from build123d import *

# Parameters (mm, degrees)
F1_DEPTH     = 22
F3_DEPTH     = 25
F4_DEPTH     = 11
F5_R         = 1.75
F6_DEPTH     = 20
F7_T1_DEPTH  = 22
F7_T6_DEPTH  = 22
F7_S7_R      = 1.75
F7_T8_DEPTH  = 14
F7_S9_R      = 1.75
F7_T10_DEPTH = 14


# Not quite as in the source:
# - a fillet or chamfer that OpenCascade refuses, or shapes differently, is made with other operations: its cross-section is extruded or revolved along the edge and cut away or added
# - after a boolean that leaves OpenCascade's solid faulty, fix() repairs it


with BuildPart() as f1:
    # F0 (on Right) → F1 (new body)
    with BuildSketch(Plane.YZ):
        with BuildLine():
            ThreePointArc((-20.9761769634, 1), (0, 21), (20.9761769634, 1))
            Line((20.9761769634, 1), (35.9761769634, 1))
            Line((35.9761769634, 1), (35.9761769634, 23))
            Line((35.9761769634, 23), (-36, 23))
            Line((-36, 23), (-36, 1))
            Line((-36, 1), (-20.9761769634, 1))
        make_face()
        with BuildLine():
            ThreePointArc((-18.973665961, -1), (-18.9934153493, -0.5001733404), (-19, 0))
            Line((-19, 0), (-21, 0))
            ThreePointArc((-21, 0), (-20.9940433961, -0.5001418641), (-20.9761769634, -1))
            Line((-20.9761769634, -1), (-18.973665961, -1))
        make_face()
        with BuildLine():
            ThreePointArc((18.973665961, 1), (1, -18.973665961), (-18.973665961, -1))
            Line((-18.973665961, -1), (-20.9761769634, -1))
            ThreePointArc((-20.9761769634, -1), (1, -20.9761769634), (20.9761769634, 1))
            Line((20.9761769634, 1), (18.973665961, 1))
        make_face()
        with BuildLine():
            ThreePointArc((-18.973665961, 1), (0, 19), (18.973665961, 1))
            Line((18.973665961, 1), (20.9761769634, 1))
            ThreePointArc((20.9761769634, 1), (0, 21), (-20.9761769634, 1))
            Line((-20.9761769634, 1), (-18.973665961, 1))
        make_face()
        with BuildLine():
            ThreePointArc((-20.9761769634, -1), (-20.9940433961, -0.5001418641), (-21, 0))
            Line((-21, 0), (-36, 0))
            Line((-36, 0), (-36, -1))
            Line((-36, -1), (-20.9761769634, -1))
        make_face()
    extrude(amount=F1_DEPTH)

    # F2 (on face) → F3 (cut)
    with BuildSketch(Plane.XY.offset(23)):
        with BuildLine():
            ThreePointArc((4.25, -24.9799919936), (6, -26.7299919936), (7.75, -24.9799919936))
            Line((7.75, -24.9799919936), (6, -24.9799919936))
            Line((6, -24.9799919936), (4.25, -24.9799919936))
        make_face()
        with BuildLine():
            Line((6, -24.9799919936), (5.93, -23.231392554))
            ThreePointArc((5.93, -23.231392554), (4.7380570536, -23.7675564283), (4.25, -24.9799919936))
            Line((4.25, -24.9799919936), (6, -24.9799919936))
        make_face()
        with BuildLine():
            Line((6, -24.9799919936), (7.75, -24.9799919936))
            ThreePointArc((7.75, -24.9799919936), (7.2124355653, -23.7180490472), (5.93, -23.231392554))
            Line((5.93, -23.231392554), (6, -24.9799919936))
        make_face()
        with BuildLine():
            ThreePointArc((17.75, -24.9799919936), (16, -23.2299919936), (14.25, -24.9799919936))
            ThreePointArc((14.25, -24.9799919936), (16, -26.7299919936), (17.75, -24.9799919936))
        make_face()
    extrude(amount=-F3_DEPTH, mode=Mode.SUBTRACT)

    # F2 (on face) → F4 (cut)
    with BuildSketch(Plane.XY.offset(23)):
        with BuildLine():
            Line((9, -24.9799919936), (7.75, -24.9799919936))
            ThreePointArc((7.75, -24.9799919936), (6, -26.7299919936), (4.25, -24.9799919936))
            Line((4.25, -24.9799919936), (3, -24.9799919936))
            ThreePointArc((3, -24.9799919936), (6, -27.9799919936), (9, -24.9799919936))
        make_face()
        with BuildLine():
            ThreePointArc((4.25, -24.9799919936), (4.7380570536, -23.7675564283), (5.93, -23.231392554))
            Line((5.93, -23.231392554), (5.88, -21.9823929544))
            ThreePointArc((5.88, -21.9823929544), (3.8366692347, -22.9015310245), (3, -24.9799919936))
            Line((3, -24.9799919936), (4.25, -24.9799919936))
        make_face()
        with BuildLine():
            ThreePointArc((5.93, -23.231392554), (7.2124355653, -23.7180490472), (7.75, -24.9799919936))
            Line((7.75, -24.9799919936), (9, -24.9799919936))
            ThreePointArc((9, -24.9799919936), (8.0784609691, -22.8166612283), (5.88, -21.9823929544))
            Line((5.88, -21.9823929544), (5.93, -23.231392554))
        make_face()
        with BuildLine():
            ThreePointArc((19, -24.9799919936), (16, -21.9799919936), (13, -24.9799919936))
            ThreePointArc((13, -24.9799919936), (16, -27.9799919936), (19, -24.9799919936))
        make_face()
        with BuildLine():
            ThreePointArc((17.75, -24.9799919936), (16, -26.7299919936), (14.25, -24.9799919936))
            ThreePointArc((14.25, -24.9799919936), (16, -23.2299919936), (17.75, -24.9799919936))
        make_face(mode=Mode.SUBTRACT)
    extrude(amount=-F4_DEPTH, mode=Mode.SUBTRACT)

    # F7: fillet of radius 10 on 2 edges, made by hand

    # F7_s2 → F7_t1 (join)
    with BuildSketch(Plane.YZ):
        with BuildLine():
            ThreePointArc((29.6647939484, 1), (23.7079599766, -0.967806711), (20.095505578, -6.0967741935))
            ThreePointArc((20.095505578, -6.0967741935), (20.8401494161, -2.5861500957), (20.9761769634, 1))
            Line((20.9761769634, 1), (29.6647939484, 1))
        make_face()
    extrude(amount=F7_T1_DEPTH)


with BuildPart() as f6:
    # F5 (on face) → F6 (new body)
    with BuildSketch(Plane(origin=(0, 0, -1), x_dir=(1, 0, 0), z_dir=(0, 0, -1))):
        Polygon((19.897114317, 27.2299919936), (16, 29.4799919936), (12.102885683, 27.2299919936), (12.102885683, 22.7299919936), (15.1405824223, 20.9761769634), (16.8594175777, 20.9761769634), (19.897114317, 22.7299919936), align=None)
        with Locations((16, 24.9799919936)):
            Circle(F5_R, mode=Mode.SUBTRACT)
    extrude(amount=F6_DEPTH)


with BuildPart() as f6b:
    # F5 (on face) → F6, piece 2 (new body)
    with BuildSketch(Plane(origin=(0, 0, -1), x_dir=(1, 0, 0), z_dir=(0, 0, -1))):
        Polygon((5.1405824223, 20.9761769634), (6.8594175777, 20.9761769634), (9.897114317, 22.7299919936), (9.897114317, 27.2299919936), (6, 29.4799919936), (2.102885683, 27.2299919936), (2.102885683, 22.7299919936), align=None)
        with Locations((6, 24.9799919936)):
            Circle(F5_R, mode=Mode.SUBTRACT)
    extrude(amount=F6_DEPTH)


with BuildPart() as f7_tool4:
    # F7_s5 → F7_t6 (new body)
    with BuildSketch(Plane.YZ):
        with BuildLine():
            ThreePointArc((-28.9827534924, -1), (-23.3031351499, -2.7694510825), (-19.6334781723, -7.4516129032))
            ThreePointArc((-19.6334781723, -7.4516129032), (-20.5594710492, -4.2788024233), (-20.9761769634, -1))
            Line((-20.9761769634, -1), (-28.9827534924, -1))
        make_face()
    extrude(amount=F7_T6_DEPTH)

    # F7_s7 → F7_t8 (cut, symmetric)
    with BuildSketch(Plane.XY.offset(-4.2)):
        with Locations((16, -24.9799919936)):
            Circle(F7_S7_R)
    extrude(amount=F7_T8_DEPTH, both=True, mode=Mode.SUBTRACT)

    # F7_s9 → F7_t10 (cut, symmetric)
    with BuildSketch(Plane.XY.offset(-4.2)):
        with Locations((6, -24.9799919936)):
            Circle(F7_S9_R)
    extrude(amount=F7_T10_DEPTH, both=True, mode=Mode.SUBTRACT)


with BuildPart() as f1_1:
    add(f1.part)

    # F7_t3: union F7_tool4
    add(f7_tool4.part)

    # F8: cut F6, F6b
    add(f6.part, mode=Mode.SUBTRACT)
    add(f6b.part, mode=Mode.SUBTRACT)

    add(f1_1.part.fix(), mode=Mode.REPLACE)


solid = f1_1.part
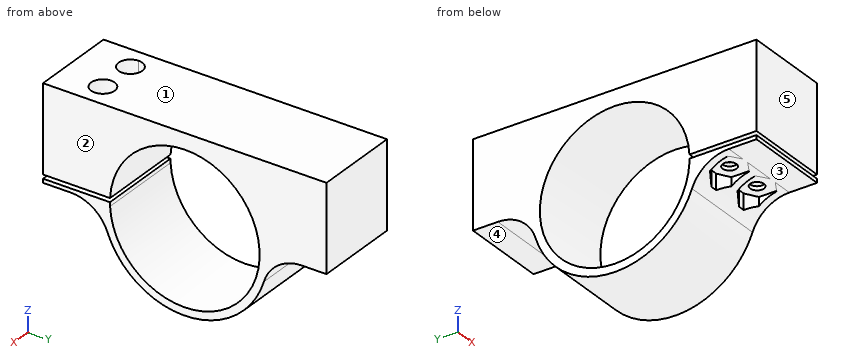
Input: part model. Units: mm. Frame: model coordinates. Face numbers are marked on the shaded views. A direction names the side the tool comes from. Coordinates: 2 decimals unless noted, no trailing zeros. Loops run counter-clockwise (first coordinate to the right, second up) from the corner with the lowest first, then second, coordinate; pieces in that order, holes last.
(1) Section B-B on x = 16. Return the cut outline in (y, z).
(2) First-contact query: pin 1 Ø3 at (x, y) = (15.5, -26) entering from +Z; pin 2 Ø1 at (x, y) = (7, -13.5) entering from -Z; pin 3 Ø7 at (x, y) = (15.5, 32) entering from -Z; pin 4 Ø2 at (x, y) = (16, -24.98) entering from +Z. Flat tips, straight axial feed; report the tip coordinate or a pass-through.
(3) Material intervals for probe 1 along Y at (x, z) = (16, 20.5); probe 2 along Y at (x, z) = (6, -0.3); probe 3 along Y at (x, z) = (5.5, 1.5), sorted ascending.
(4) Section D-D on z = -18. Return the cut outline in (x, y), then the cut area to 3 significant figures.
(5) Section A-A on z = 2. Return the cut outline in (x, y), then the cut area to 3 significant figures.
(6) Pull-direction query (X, two-part tool) for the marked faces 1, 2 and 3; classes: released by +X, released by -X, zero draft, split by the parting line, or undercut.
(7) Section C-C on y = -15. Return the cut outline in (x, z), then the cut area to 3 significant figures.
(8) Set-up query: the marked faces 4 and 5. Return all of +Z, -Z, +X, -X, +Y, -Y with unobstructed straight access to the full face (end or side cutting, diameter ignored); none if empty.
Data:
1. outline: (-36, -1) - (-26.73, -1) - (-26.73, 0) - (-36, 0) - close; (-36, 1) - (-26.73, 1) - (-26.73, 12) - (-27.98, 12) - (-27.98, 23) - (-36, 23) - close; (-23.23, -1) - (-20.98, -1) - (-20.98, -5.01) arc R10 cw to (-19.63, -7.45) arc R21 ccw to (20.1, -6.1) arc R10 cw to (29.66, 1) - (35.98, 1) - (35.98, 23) - (-21.98, 23) - (-21.98, 12) - (-23.23, 12) - (-23.23, 1) - (-18.97, 1) arc R19 cw (long way) to (-19, 0) - (-23.23, 0) - close
2. pin 1: stops at z = 12
2. pin 2: stops at z = -16.49
2. pin 3: stops at z = 0.93
2. pin 4: passes through
3. probe 1: y = -36 to -27.98, -21.98 to 35.98
3. probe 2: y = -36 to -26.73, -23.23 to -19, 19 to 24.73
3. probe 3: y = -36 to -26.66, -23.3 to -18.94, 18.94 to 35.98
4. outline: (0, -10.82) - (22, -10.82) - (22, -6.08) - (0, -6.08) - close; (0, 6.08) - (22, 6.08) - (22, 10.82) - (0, 10.82) - close
4. area: 208 mm2
5. outline: (0, -36) - (22, -36) - (22, -18.89) - (0, -18.89) - close; (0, 18.89) - (22, 18.89) - (22, 35.98) - (0, 35.98) - close; hole circle Ø3.5 at (6, -24.98); hole circle Ø3.5 at (16, -24.98)
5. area: 733 mm2
6. face 1: zero draft
6. face 2: released by +X
6. face 3: undercut
7. outline: (0, -14.7) - (22, -14.7) - (22, -11.66) - (0, -11.66) - close; (0, 11.66) - (22, 11.66) - (22, 23) - (0, 23) - close
7. area: 316 mm2
8. face 4: -Z, +X, -X, +Y
8. face 5: +Z, -Z, +X, -X, -Y
